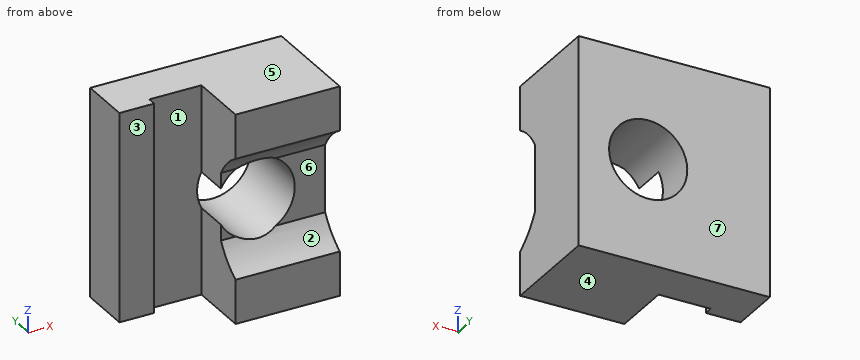
```python
from build123d import *

# Parameters (mm, degrees)
BOSS_EXTRUDE1_DEPTH      = 4
BOSS_EXTRUDE1_DEPTH_BACK = 7
CUT_EXTRUDE1_DEPTH       = 12
CUT_EXTRUDE1_DEPTH_BACK  = 12
SKETCH3_R                = 2.25
CUT_EXTRUDE2_DEPTH       = 12


with BuildPart() as part:
    # Sketch1 → Boss-Extrude1 (new, two sides: drawn at the far end of the back side and taken through both)
    with BuildSketch(Plane(origin=(0, 0, 0), x_dir=(0, 0, -1), z_dir=(1, 0, 0)).offset(-BOSS_EXTRUDE1_DEPTH_BACK)):
        with BuildLine():
            Line((6, -6), (6, 0))
            Line((6, 0), (-6, 0))
            Line((-6, 0), (-6, -6))
            Line((-6, -6), (-3.464101615, -6))
            ThreePointArc((-3.464101615, -6), (-2.802517077, -5.145898034), (-1.936491673, -4.5))
            Line((-1.936491673, -4.5), (1.936491673, -4.5))
            ThreePointArc((1.936491673, -4.5), (2.802517077, -5.145898034), (3.464101615, -6))
            Line((3.464101615, -6), (6, -6))
        make_face()
    extrude(amount=BOSS_EXTRUDE1_DEPTH + BOSS_EXTRUDE1_DEPTH_BACK)

    # Sketch2 → Cut-Extrude1 (cut, two sides: drawn at the far end of the back side and taken through both)
    with BuildSketch(Plane.XY.offset(-CUT_EXTRUDE1_DEPTH_BACK)):
        Polygon((-7, -3), (-5, -3), (-5, -2.5), (-2, -2.5), (-2, -6), (-7, -6), align=None)
    extrude(amount=CUT_EXTRUDE1_DEPTH + CUT_EXTRUDE1_DEPTH_BACK, mode=Mode.SUBTRACT)

    # Sketch3 → Cut-Extrude2 (cut, through all)
    with BuildSketch(Plane(origin=(0, 0, 0), x_dir=(1, 0, 0), z_dir=(0, 1, 0))):
        with Locations(Location((0, 0, 0), (0, 0, 270))):
            Circle(SKETCH3_R)
    extrude(amount=-CUT_EXTRUDE2_DEPTH, mode=Mode.SUBTRACT)


solid = part.part
```
Input: part model. Units: mm. Frame: model coordinates. Face numbers are marked on the shaded views. A direction names the side the tool comes from. Give positions to 0.01 mm unless a question says otherwise; leave off trailing zeros. Order: outer loops, then holes, each group sorted by start corner. A loop starts at its lowest first (then second) coordinate and runs counter-clockwise, first axis right, second up.
1. Line query: probe 1 along X at (y, z) = (-0.5, 0); probe 2 along Z at (x, y) = (0, -2.05); probe 3 along Y at (x, z) = (-4.5, -3.75). Output: solid intervals per line, ascending.
Computed:
probe 1: x = -7 to -2.25, 2.25 to 4
probe 2: z = -6 to -2.25, 2.25 to 6
probe 3: y = -2.5 to 0
2. Cut plane D-D (z = 4.75). Return loops of the section in (x, y), and give its area (3 significant figures).
Computed:
outline: (-7, -3) - (-5, -3) - (-5, -2.5) - (-2, -2.5) - (-2, -6) - (4, -6) - (4, 0) - (-7, 0) - close
area: 49.5 mm2
3. Pin query (flat end, axial travel): pin 1 Ø2 at (x, y) = (-3.5, -4) entering from -Z; pin 2 Ø1 at (x, z) = (-6.5, -2) entering from -Y; pin 3 Ø0.9 at (x, z) = (-4, -1) entering from -Y; pin 4 Ø1 at (y, z) = (-4, -4) entering from -X. Return the tip coordinate at first contact, or that it passes through.
Computed:
pin 1: passes through
pin 2: stops at y = -3
pin 3: stops at y = -2.5
pin 4: stops at x = -2
4. Set-up query: the marked faces 1, 2 and 3. Return all of +Z, -Z, +X, -X, +Y, -Y with unobstructed straight access to the full face (end or side cutting, diameter ignored); none if empty.
Computed:
face 1: +Z, -Z, -Y
face 2: +X, -X, -Y
face 3: +Z, -Z, -X, -Y
5. Cut plane C-C (y = -5). Return loops of the section in (x, z), and give its area (3 significant figures).
Computed:
outline: (-2, -6) - (4, -6) - (4, -2.65) - (-2, -2.65) - close; (-2, 2.65) - (4, 2.65) - (4, 6) - (-2, 6) - close
area: 40.3 mm2
6. Cut plane B-B (z = 0). Return loops of the section in (x, y).
Computed:
outline: (-7, -3) - (-5, -3) - (-5, -2.5) - (-2.25, -2.5) - (-2.25, 0) - (-7, 0) - close; (2.25, -4.5) - (4, -4.5) - (4, 0) - (2.25, 0) - close
7. Draft query along Z for the marked faces 4, 5, 6 and 7. Return one class per face: released by +Z, released by -Z, zero draft, split by the parting line, or undercut.
Computed:
face 4: released by -Z
face 5: released by +Z
face 6: undercut
face 7: zero draft
8. Cut plane A-A (x = 0). Return loops of the section in (y, z), and give its area (3 significant figures).
Computed:
outline: (-6, -6) - (0, -6) - (0, -2.25) - (-4.69, -2.25) arc R4 cw to (-6, -3.46) - close; (-6, 3.46) arc R4 cw to (-4.69, 2.25) - (0, 2.25) - (0, 6) - (-6, 6) - close
area: 43.2 mm2
